Geometry: final body of the model. Coordinates: model frame, mm. Face numbers are marked on the shaded views. A direction names the side the tool comes from. Give positions to 0.01 mm unless a question says otherwise; leave off trailing zeros. Write each loop counter-clockwise with the first axis right and the second up, starting at its lowest first coordinate (ties: lowest second). Pieces come first, ordered by that corner, then holes.
Autodesk Inventor part; units mm, degrees
ref_plane "YZ Plane" through (0, 0, 0) normal (1, 0, 0) x (0, 1, 0)
ref_plane "XZ Plane" through (0, 0, 0) normal (0, 1, 0) x (-1, 0, 0)
ref_plane "XY Plane" through (0, 0, 0) normal (0, 0, 1) x (1, 0, 0)
sketch "Boceto1" plane through (0, 0, 0) normal (0, 0, 1) x (1, 0, 0)
  line L0 (0, 21.3006) -> (0, 0)
  line L1 (0, 15.4538) -> (5, 15.4538)
  line L2 (5, 15.4538) -> (5, 7.4538)
  line L3 (5, 7.4538) -> (0, 7.4538)
  line L4 (7, 7.4538) -> (5, 7.4538)
  line L5 (7, 7.4538) -> (7, 2.4538)
  line L6 (7, 2.4538) -> (0, 2.4538)
  line L7 (3, 2.4538) -> (3, 0.9538)
  line L8 (2, 15.4538) -> (2, -0.5462)
  line L9 (3, -0.5462) -> (2, -0.5462)
  line L10 (0, 0.6254) -> (0, -1.387)
  line L11 (3, -0.5462) -> (3, -0.5462)
  arc A0 (6, 2.4538) -> (3, -0.5462) centre (6, -0.5462) ccw
  line L12 (3, 0.9538) -> (3, -0.5462)
  point P0 (2, 2.4538)
  point P1 (2, 7.4538)
  dimension "d0" = 10
  dimension "d1" = 4
  dimension "d2" = 14
  dimension "d4" = 5
  dimension "d6" = 8
  dimension "d9" = 15.4538
  dimension "d10" = 13.8468
  dimension "d11" = 1.8283
  dimension "d12" = 3.8408
  dimension "d16" = 3
  dimension "d17" = 1
  dimension "d18" = 4
  dimension "d19" = 0.5462
  dimension "d20" = 6
  dimension "d21" = 1
revolve "Revolución1" add sketch "Boceto1" angle 360 about axis through (0, 21.3006, 0) along (0, -1, 0) contours L1 L2 L3 L8 | L3 L4 L5 L6 L8 | L6 L7 L12 L9 L8
revolve "Revolución2" add sketch "Boceto1" angle 360 about axis through (0, 0.6254, 0) along (0, -1, 0) contours L6 A0 L12 L7
sketch "Boceto2" plane through (0, 7.4538, 0) normal (0, 1, 0) x (1, 0, 0)
  line L0 (0, 11.3393) -> (0, -11.3393) construction
  line L1 (-23.3185, 0) -> (23.3185, 0) construction
  line L2 (7, 4.5) -> (7, -4.5)
  line L3 (-7, 4.5) -> (-7, -4.5)
  circle A0 centre (0, 0) radius 7
  line L4 (-7, 4.5) -> (0, 7)
  line L5 (0, 7) -> (7, 4.5)
  line L6 (-7, -4.5) -> (0, -7)
  line L7 (7, -4.5) -> (0, -7)
  arc A1 (0, 7) -> (-4.4344, 5.4163) centre (0, 0) ccw
  arc A2 (4.4344, 5.4163) -> (0, 7) centre (0, 0) ccw
  arc A3 (0, -7) -> (4.4344, -5.4163) centre (0, 0) ccw
  arc A4 (-4.4344, -5.4163) -> (0, -7) centre (0, 0) ccw
  point P0 (7, 0)
  point P1 (-7, 0)
  point P2 (0, -7)
  point P3 (0, -7)
  point P4 (0, 7)
  point P5 (0, 7)
  point P6 (7, 0)
  point P7 (-7, 0)
  dimension "d24" = 9
  dimension "d26" = 9
  dimension "d27" = 7
  dimension "d28" = 7
extrude "Extrusión1" cut sketch "Boceto2" against normal through all contours A0 L7 | A0 L6
extrude "Extrusión2" cut sketch "Boceto2" against normal through all contours L5 A0 | L4 A0
extrude "Extrusión3" add sketch "Boceto2" against normal blind 5 contours L2 A0 L5 | L2 L7 A0 | A0 L3 L4 | L6 L3 A0
thread "Rosca1"
properties part number "1-HUDSON-8-30-TDR HAND PUMP BODY BOTTOM INLET"
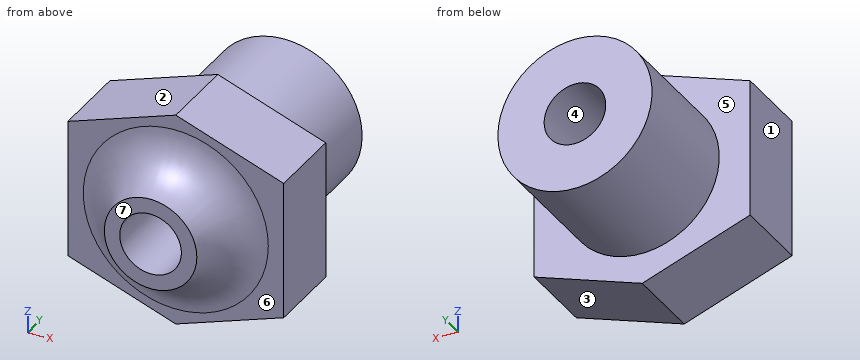
Q1. Pin query (flat end, axial travel): P1, Ø4, axis at x = -3.5, y = 4.5, coming from the +Z side; P2, Ø4, axis at y = 13, z = 5.5, coming from the -X side; P3, Ø3, axis at x = -0.5, y = 10.5, coming from the +Z side. Return the tip coordinate at first contact, or that it passes through.
Filled sheet:
P1: stops at z = 6.46
P2: stops at x = -3.57
P3: stops at z = 5
Q2. Section C-C on y = 8.5. Output: boundary loops of the cut face in (x, z).
Filled sheet:
outline: circle Ø10 at (0, 0); hole circle Ø4 at (0, 0)
Q3. Pull-direction query (Z, two-part tool) for the marked faces 1, 2, 3 and 4; classes: released by +Z, released by -Z, zero draft, split by the parting line, or undercut.
Filled sheet:
face 1: zero draft
face 2: released by +Z
face 3: released by -Z
face 4: undercut
Q4. Section B-B on z = 0. Output: boundary loops of the cut face in (x, y).
Filled sheet:
outline: (-7, 2.45) - (-6, 2.45) arc R3 cw to (-3, -0.55) - (-2, -0.55) - (-2, 15.45) - (-5, 15.45) - (-5, 7.45) - (-7, 7.45) - close; (2, -0.55) - (3, -0.55) arc R3 cw to (6, 2.45) - (7, 2.45) - (7, 7.45) - (5, 7.45) - (5, 15.45) - (2, 15.45) - close
Q5. Access query for the marked faces 5, 6 and 7. Directions: +Z, -Z, +X, -X, +Y, -Y. A direction counts if a zero-diameter tool reaches every point of the face in a straight line with its end or side. Return the directions, or none.
Filled sheet:
face 5: +Y
face 6: -Y
face 7: +Z, -Z, +X, -X, -Y
Q6. Section A-A on y = 4.75. Output: boundary loops of the cut face in (x, z).
Filled sheet:
outline: (-7, -4.5) - (0, -7) - (7, -4.5) - (7, 4.5) - (0, 7) - (-7, 4.5) - close; hole circle Ø4 at (0, 0)
Q7. Ray query, line 1 along Z through (x, y) = (0, 6); line 2 along Z through (x, y) = (0, 10.75); line 3 along Y through (x, z) = (-5.5, 3.75). Return the intervals inside material, ascending.
Filled sheet:
line 1: z = -7 to -2, 2 to 7
line 2: z = -5 to -2, 2 to 5
line 3: y = 2.45 to 7.45
